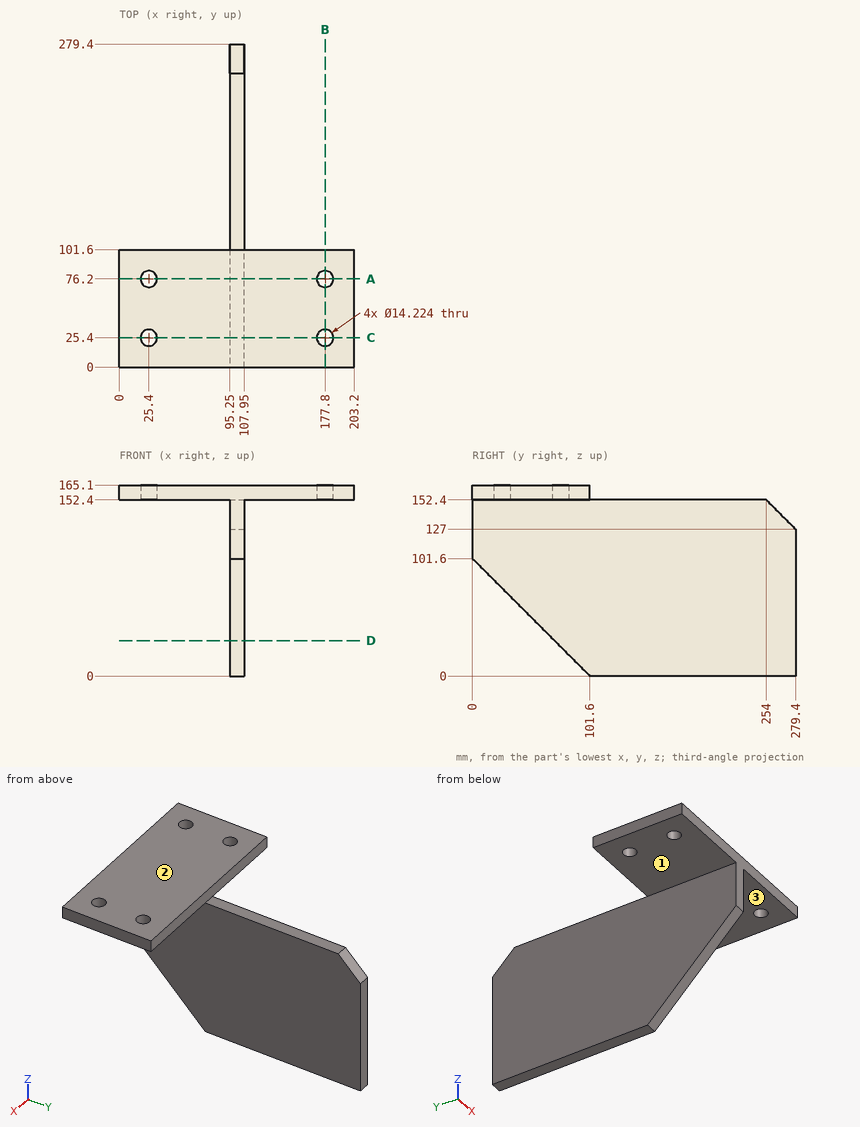
For this review, use the dimensioned drawing (mm, ordinates from the lowest corner) and the shaded views. A direction names the side the tool comes from. Coordinates: 2 decimals unless noted, no trailing zeros. Write each loop counter-clockwise with the first axis right and the second up, starting at its lowest first coordinate (ties: lowest second). Pieces come first, ordered by that corner, then holes. Notation, with made-up numbers: (36.25, 52) - (93.25, 52) arc R15 cw to (93.25, 69) - close; hole circle Ø3 at (16.5, 53). An arc over 180 degrees is marked (long way). One line per item, written item: value.
1) Add section A-A (y = 76.2). State the section outline as (x, z) points, plus the area to 3 significant figures.
Answer sheet:
outline: (0, 152.4) - (18.29, 152.4) - (18.29, 165.1) - (0, 165.1) - close; (32.51, 152.4) - (95.25, 152.4) - (95.25, 25.4) - (107.95, 25.4) - (107.95, 152.4) - (170.69, 152.4) - (170.69, 165.1) - (32.51, 165.1) - close; (184.91, 152.4) - (203.2, 152.4) - (203.2, 165.1) - (184.91, 165.1) - close
area: 3,830 mm2
2) Add section D-D (z = 30.5). State the section outline as (x, y) points.
Answer sheet:
outline: (95.25, 71.1) - (107.95, 71.1) - (107.95, 279.4) - (95.25, 279.4) - close
3) Add section C-C (y = 25.4). State the section outline as (x, z) points, plus the area to 3 significant figures.
Answer sheet:
outline: (0, 152.4) - (18.29, 152.4) - (18.29, 165.1) - (0, 165.1) - close; (32.51, 152.4) - (95.25, 152.4) - (95.25, 76.2) - (107.95, 76.2) - (107.95, 152.4) - (170.69, 152.4) - (170.69, 165.1) - (32.51, 165.1) - close; (184.91, 152.4) - (203.2, 152.4) - (203.2, 165.1) - (184.91, 165.1) - close
area: 3,190 mm2
4) For the marked faces 1, 2 and 3, list the 3-axis set-ups (+Z, -Z, +X, -X, +Y, -Y) from which the entire face can be reached by the end or side of a thin tool; tool diameter is ignored.
Answer sheet:
face 1: -Z, -X, +Y, -Y
face 2: +Z, +X, -X, +Y, -Y
face 3: -Z, +X, +Y, -Y
5) Add section B-B (x = 177.8). State the section outline as (y, z) points, plus the area to 3 significant figures.
Answer sheet:
outline: (0, 152.4) - (18.29, 152.4) - (18.29, 165.1) - (0, 165.1) - close; (32.51, 152.4) - (69.09, 152.4) - (69.09, 165.1) - (32.51, 165.1) - close; (83.31, 152.4) - (101.6, 152.4) - (101.6, 165.1) - (83.31, 165.1) - close
area: 929 mm2
6) Insertion check: pin 1 (16.5 mm diameter, centred on x = 25.4, y = 76.2, fed in from +Z); pin 2 (11.5 mm diameter, centred on x = 177.8, y = 25.4, fed in from -Z); pin 3 (6 mm diameter, centred on y = 244.5, z = 84, fed in from +X); pin 4 (10 mm diameter, centred on y = 110.5, z = 45, fed in from -X). Each pin has a flat end and moves straight along its axis. Give the tip position at first contact, or say it passes through.
Answer sheet:
pin 1: stops at z = 165.1
pin 2: passes through
pin 3: stops at x = 107.95
pin 4: stops at x = 95.25
7) To check wall thickness, follow probe 1 along Y at (x, z) = (177.8, 158); probe 2 along Y at (x, z) = (139, 158.5); probe 3 along X at (y, z) = (262.5, 106.5). State the ranges of each line that lie inside material, in increasing order.
Answer sheet:
probe 1: y = 0 to 18.29, 32.51 to 69.09, 83.31 to 101.6
probe 2: y = 0 to 101.6
probe 3: x = 95.25 to 107.95
